Job drawing, mm, ordinate dimensions from the low corner. One solid piece. Give positions to 0.01 mm unless a question says otherwise; leave off trailing zeros. Loops run counter-clockwise (first coordinate to the right, second up) from the corner with the lowest first, then second, coordinate; pieces in that order, holes last. Notation, with made-up numbers: M 15.25,71.5 L 60.25,71.5 A7 ccw 60.25,75.5 Z; hole C 31.5,-10 d1. An arc over 180 degrees is marked long. Answer as CSV lines item,"result".
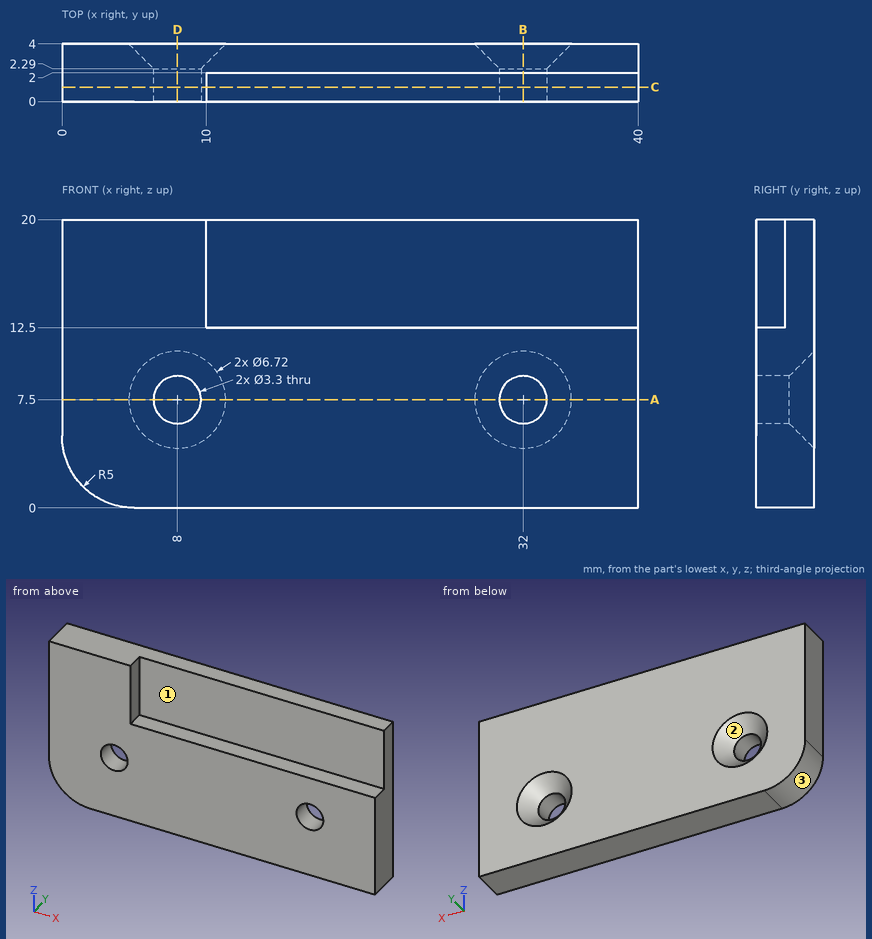
1) Mould opens along X. For the marked faces 1, 2 and 3 say: +X half, -X half, draft (parallel to the pull), parting line (faces both ways), or undercut.
Answer below:
face 1,"draft"
face 2,"undercut"
face 3,"-X half"
2) Band-saw the part on A-A on z = 7.5. Give the cut face in (x, y), and give its area (3 significant figures).
Answer below:
outline,"M 0,0 L 6.35,0 L 6.35,2.29 L 4.64,4 L 0,4 Z; M 9.65,0 L 30.35,0 L 30.35,2.29 L 28.64,4 L 11.36,4 L 9.65,2.29 Z; M 33.65,0 L 40,0 L 40,4 L 35.36,4 L 33.65,2.29 Z"
area,"128 mm^2"
3) Drill centre lines: line 1 (X direction, y = 1.8, z = 7.5); line 2 (Z direction, x = 32, y = 1.15); line 3 (X direction, y = 2.5, z = 7.5). Where is each one in solid material? Low to high. Write a range as from..to.
Answer below:
line 1,"x = 0..6.35, 9.65..30.35, 33.65..40"
line 2,"z = 0..5.85, 9.15..12.5"
line 3,"x = 0..6.14, 9.86..30.14, 33.86..40"
4) Band-saw the part on D-D on x = 8. Give the cut face in (y, z), and give its area (3 significant figures).
Answer below:
outline,"M 0,0 L 4,0 L 4,4.14 L 2.29,5.85 L 0,5.85 Z; M 0,9.15 L 2.29,9.15 L 4,10.86 L 4,20 L 0,20 Z"
area,"63.9 mm^2"
5) Flat gauge pins, fed straight in: pin 1 (0.6 mm diameter, centred on y = 1.5, z = 17.5, fed in from +X); pin 2 (4.5 mm diameter, centred on x = 8, z = 7.5, fed in from +Y); pin 3 (0.6 mm diameter, centred on x = 18.5, y = 0.5, fed in from +Z). Where does each tip first touch, or does it go through?
Answer below:
pin 1,"stops at x = 10"
pin 2,"stops at y = 2.89"
pin 3,"stops at z = 12.5"
6) Band-saw the part on C-C on y = 1. Give the cut face in (x, z), and give its area (3 significant figures).
Answer below:
outline,"M 0,5 A5 ccw 5,0 L 40,0 L 40,12.5 L 10,12.5 L 10,20 L 0,20 Z; hole C 8,7.5 d3.3; hole C 32,7.5 d3.3"
area,"553 mm^2"
7) Band-saw the part on B-B on x = 32. Give the cut face in (y, z), and give its area (3 significant figures).
Answer below:
outline,"M 0,0 L 4,0 L 4,4.14 L 2.29,5.85 L 0,5.85 Z; M 0,9.15 L 2.29,9.15 L 4,10.86 L 4,20 L 2,20 L 2,12.5 L 0,12.5 Z"
area,"48.9 mm^2"
